from build123d import *

# Parameters (mm, degrees)
CYLINDER1875_R     = 1.6
CYLINDER1875_DEPTH = 80
CYLINDER1873_R     = 1.6
CYLINDER1873_DEPTH = 80
CYLINDER1874_R     = 1.6
CYLINDER1874_DEPTH = 80
CYLINDER1872_R     = 1.6
CYLINDER1872_DEPTH = 80
CYLINDER1871_R     = 6
CYLINDER1871_DEPTH = 20
BOX745_W           = 26
BOX745_H           = 3
BOX745_DEPTH       = 36


with BuildPart() as obj1:
    # Cylinder1875 → Cylinder1875 (new body)
    with BuildSketch(Plane(origin=(-10, 80, 31), x_dir=(1, 0, 0), z_dir=(0, -1, 0))):
        Circle(CYLINDER1875_R)
    extrude(amount=CYLINDER1875_DEPTH)


with BuildPart() as obj2:
    # Cylinder1873 → Cylinder1873 (new body)
    with BuildSketch(Plane(origin=(10, 80, 55), x_dir=(1, 0, 0), z_dir=(0, -1, 0))):
        Circle(CYLINDER1873_R)
    extrude(amount=CYLINDER1873_DEPTH)


with BuildPart() as obj3:
    # Cylinder1874 → Cylinder1874 (new body)
    with BuildSketch(Plane(origin=(10, 80, 31), x_dir=(1, 0, 0), z_dir=(0, -1, 0))):
        Circle(CYLINDER1874_R)
    extrude(amount=CYLINDER1874_DEPTH)


with BuildPart() as compound844:
    # Cylinder1872 → Cylinder1872 (new body)
    with BuildSketch(Plane(origin=(-10, 80, 55), x_dir=(1, 0, 0), z_dir=(0, -1, 0))):
        Circle(CYLINDER1872_R)
    extrude(amount=CYLINDER1872_DEPTH)

    # Compound844: union obj1, obj2, obj3
    add(obj1.part)
    add(obj2.part)
    add(obj3.part)


with BuildPart() as compound844_1:
    # Compound844 placement: moved
    add(compound844.part.moved(Location((0, -90, -141))))


with BuildPart() as obj4:
    # Cylinder1871 → Cylinder1871 (new body)
    with BuildSketch(Plane(origin=(0, -60, -98), x_dir=(1, 0, 0), z_dir=(0, -1, 0))):
        Circle(CYLINDER1871_R)
    extrude(amount=CYLINDER1871_DEPTH)


with BuildPart() as cut683:
    # Box745 → Box745 (new body)
    with BuildSketch(Plane(origin=(-13, -72, -116), x_dir=(1, 0, 0), z_dir=(0, 0, 1))):
        with Locations((13, 1.5)):
            Rectangle(BOX745_W, BOX745_H)
    extrude(amount=BOX745_DEPTH)

    # Cut682: cut obj4
    add(obj4.part, mode=Mode.SUBTRACT)

    # Cut683: cut Compound844
    add(compound844_1.part, mode=Mode.SUBTRACT)


solid = cut683.part
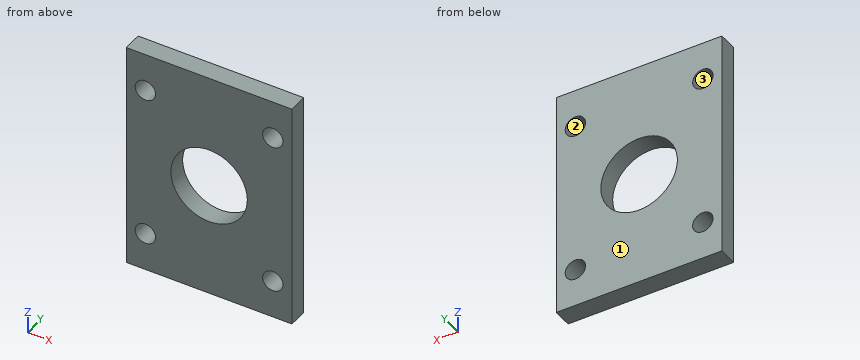
Geometry: final body of the model. Coordinates: model frame, mm. Face numbers are marked on the shaded views. Coordinates: 2 decimals unless noted, no trailing zeros. Loops run counter-clockwise (first coordinate to the right, second up) from the corner with the lowest first, then second, coordinate; pieces in that order, holes last. Notation, with made-up numbers: (38, 23.25) - (62, 23.25) arc R21 cw to (62, 59.25) - close; hole circle Ø1 at (29, -0.75). An arc over 180 degrees is marked (long way). Put each result on its own line as item: value. Start each with the question number.
Q1. Cut plane B-B, the plane x = 0. Return loops of the section in (y, z), and give its area (3 significant figures).
Q2. Cut plane C-C, the plane z = -110. Return loops of the section in (x, y), and give its area (3 significant figures).
Q3. Pull-direction query (X, two-part tool) for the marked faces 1, 2 and 3; classes: released by +X, released by -X, zero draft, split by the parting line, or undercut.
Q4. Line query: line 1 (X direction, y = -70.5, z = -110); line 2 (Z direction, x = 10, y = -70.95); line 3 (Z direction, x = 0.25, y = -71.65). Output: solid intervals per line, ascending.
Q5. Pin query (flat end, axial travel): pin 1 Ø9.5 at (x, z) = (0, -98) entering from -Y. Return the tip coordinate at first contact, or that it passes through.
Q6. Cut plane D-D, the plane y = -69.9. Return loops of the section in (x, z).
Q7. Cut plane A-A, the plane z = -98. Return loops of the section in (x, y), and give its area (3 significant figures).
Filled sheet:
1. outline: (-72, -116) - (-69, -116) - (-69, -104) - (-72, -104) - close; (-72, -92) - (-69, -92) - (-69, -80) - (-72, -80) - close
1. area: 72.0 mm²
2. outline: (-13, -72) - (-11.6, -72) - (-11.6, -69) - (-13, -69) - close; (-8.4, -72) - (8.4, -72) - (8.4, -69) - (-8.4, -69) - close; (11.6, -72) - (13, -72) - (13, -69) - (11.6, -69) - close
2. area: 58.8 mm²
3. face 1: zero draft
3. face 2: undercut
3. face 3: undercut
4. line 1: -13 to -11.6, -8.4 to 8.4, 11.6 to 13
4. line 2: -116 to -111.6, -108.4 to -87.6, -84.4 to -80
4. line 3: -116 to -103.99, -92.01 to -80
5. pin 1: through
6. outline: (-13, -116) - (13, -116) - (13, -80) - (-13, -80) - close; hole circle Ø3.2 at (-10, -110); hole circle Ø3.2 at (-10, -86); hole circle Ø12 at (0, -98); hole circle Ø3.2 at (10, -110); hole circle Ø3.2 at (10, -86)
7. outline: (-13, -72) - (-6, -72) - (-6, -69) - (-13, -69) - close; (6, -72) - (13, -72) - (13, -69) - (6, -69) - close
7. area: 42.0 mm²
